Part model, mm, in its own coordinate system. Round coordinates to 2 decimals unless told otherwise and drop trailing zeros. Loops run counter-clockwise (first coordinate to the right, second up) from the corner with the lowest first, then second, coordinate; pieces in that order, holes last. Notation, with made-up numbers: M 78,51.5 L 98,51.5 A27 cw 98,86.5 Z; hole C 19.5,72.25 d7. An arc over 180 degrees is marked long. Put each result on its own line as item: value. Start each with the question number.
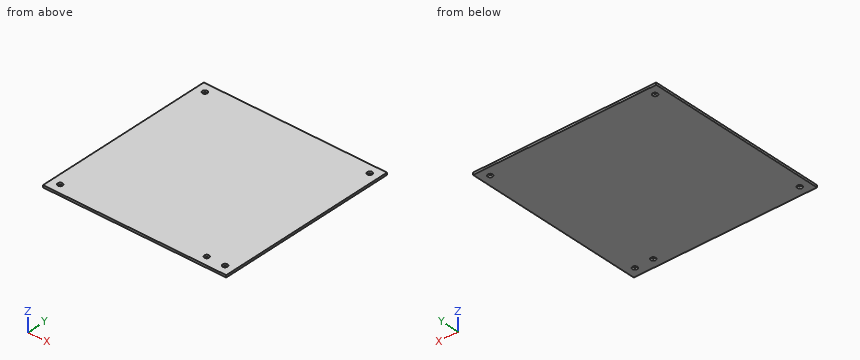
Autodesk Inventor part; units mm, degrees
ref_plane "YZ Plane" through (0, 0, 0) normal (1, 0, 0) x (0, 1, 0)
ref_plane "XZ Plane" through (0, 0, 0) normal (0, 1, 0) x (-1, 0, 0)
ref_plane "XY Plane" through (0, 0, 0) normal (0, 0, 1) x (1, 0, 0)
sketch "Sketch1" plane through (0, 0, 0) normal (0, 0, 1) x (1, 0, 0)
  line L0 (-127, -127) -> (127, -127)
  line L1 (127, -127) -> (127, 127)
  line L2 (127, 127) -> (-127, 127)
  line L3 (-127, 127) -> (-127, -127)
  line L4 (-127, -127) -> (127, 127) construction
  point P0 (0, 0)
  point P1 (0, 0)
  dimension "d0" = 254
  dimension "d1" = 254
extrude "Extrusion1" add sketch "Sketch1" along normal blind 3
sketch "Sketch2" plane through (0, 0, 3) normal (0, 0, 1) x (1, 0, 0)
  line L0 (-114.3, -114.3) -> (114.3, -114.3) construction
  line L1 (114.3, -114.3) -> (114.3, 114.3) construction
  line L2 (114.3, 114.3) -> (-114.3, 114.3) construction
  line L3 (-114.3, 114.3) -> (-114.3, -114.3) construction
  line L4 (-114.3, -114.3) -> (114.3, 114.3) construction
  point P0 (0, 0)
  point P1 (0, 0)
  point P2 (88.9, -114.3)
  dimension "d4" = 228.6
  dimension "d5" = 228.6
hole "Hole1" at (-114.3, 114.3, 3) at (114.3, 114.3, 3) at (114.3, -114.3, 3) at (-114.3, -114.3, 3) direction (0, 0, -1) diameter 6.7564 end through all
sketch "Sketch3" plane through (0, 0, 3) normal (0, 0, 1) x (1, 0, 0)
  point P0 (0, 0)
  point P1 (88.9, -114.3)
hole "Hole2" at (88.9, -114.3, 3) direction (0, 0, -1) diameter 6.7564 depth 25.4 tip angle 118
1. Wall check: L1, parallel to Y at x = 114.3, z = 1.95; L2, parallel to X at y = -114.3, z = 1.5. Give the ranges that are in metal, low to high.
2. Cut at A-A, the plane y = 114.3. Give the cut face in (x, z), and give its area (3 significant figures).
3. Cut at B-B, the plane x = 88.9. Give the cut face in (y, z).
4. Drop a flat-ended pin along its axis: pin 1 (6 mm diameter, centred on x = 88.9, y = -114.3, fed in from -Z). Give the stop position or say it passes through.
Results list:
1. L1: y = -127 to -117.68, -110.92 to 110.92, 117.68 to 127
1. L2: x = -127 to -117.68, -110.92 to 85.52, 92.28 to 110.92, 117.68 to 127
2. outline: M -127,0 L -117.68,0 L -117.68,3 L -127,3 Z; M -110.92,0 L 110.92,0 L 110.92,3 L -110.92,3 Z; M 117.68,0 L 127,0 L 127,3 L 117.68,3 Z
2. area: 721 mm^2
3. outline: M -127,0 L -117.68,0 L -117.68,3 L -127,3 Z; M -110.92,0 L 127,0 L 127,3 L -110.92,3 Z
4. pin 1: passes through
